```python
from build123d import *

# Parameters (mm, degrees)
SKETCH1_R           = 2.25
BOSS_EXTRUDE1_DEPTH = 2.6
SKETCH2_R           = 4.75
SKETCH2_R_2         = 2.5
BOSS_EXTRUDE2_DEPTH = 4.5
CHAMFER1_SIZE       = 0.75
SKETCH3_R           = 3.75
BOSS_EXTRUDE3_DEPTH = 3
CHAMFER2_SIZE       = 0.3
CHAMFER3_SIZE       = 0.5


with BuildPart() as part:
    # Sketch1 → Boss-Extrude1 (new body)
    with BuildSketch(Plane(origin=(0, 0, 0), x_dir=(0, 0, -1), z_dir=(1, 0, 0))):
        with BuildLine():
            Line((-21, -10), (6, -10))
            ThreePointArc((6, -10), (8.828427125, -8.828427125), (10, -6))
            Line((10, -6), (10, 19))
            ThreePointArc((10, 19), (8.828427125, 21.828427125), (6, 23))
            Line((6, 23), (-9.695652174, 23))
            ThreePointArc((-9.695652174, 23), (-11.354136506, 22.63997661), (-12.714074263, 21.62471486))
            Line((-12.714074263, 21.62471486), (-24.018422089, 8.62471486))
            ThreePointArc((-24.018422089, 8.62471486), (-24.746577662, 7.401126626), (-25, 6))
            Line((-25, 6), (-25, -6))
            ThreePointArc((-25, -6), (-23.828427125, -8.828427125), (-21, -10))
        make_face()
        with Locations((-15, 0)):
            Circle(SKETCH1_R, mode=Mode.SUBTRACT)
        with Locations((0, 17.25)):
            Circle(SKETCH1_R, mode=Mode.SUBTRACT)
        Circle(SKETCH1_R, mode=Mode.SUBTRACT)
    extrude(amount=BOSS_EXTRUDE1_DEPTH)

    # Sketch2 → Boss-Extrude2 (add)
    with BuildSketch(Plane.ZY):
        with Locations(Location((0, 17.25, 0), (0, 0, 180))):
            Circle(SKETCH2_R)
        with Locations((0, 17.25)):
            Circle(SKETCH2_R_2, mode=Mode.SUBTRACT)
    extrude(amount=BOSS_EXTRUDE2_DEPTH)

    # Chamfer1
    chamfer1_edges = [part.edges().sort_by_distance(p)[0] for p in [
        (-4.5, 17.25, 4.75),
    ]]
    chamfer(chamfer1_edges, length=CHAMFER1_SIZE)

    # Sketch3 → Boss-Extrude3 (add)
    with BuildSketch(Plane(origin=(2.6, 0, 0), x_dir=(0, 0, -1), z_dir=(1, 0, 0))):
        with BuildLine():
            Line((-21, -10), (6, -10))
            ThreePointArc((6, -10), (8.828427125, -8.828427125), (10, -6))
            Line((10, -6), (10, 19))
            ThreePointArc((10, 19), (8.828427125, 21.828427125), (6, 23))
            Line((6, 23), (-9.695652174, 23))
            ThreePointArc((-9.695652174, 23), (-11.354136506, 22.63997661), (-12.714074263, 21.62471486))
            Line((-12.714074263, 21.62471486), (-24.018422089, 8.62471486))
            ThreePointArc((-24.018422089, 8.62471486), (-24.746577662, 7.401126626), (-25, 6))
            Line((-25, 6), (-25, -6))
            ThreePointArc((-25, -6), (-23.828427125, -8.828427125), (-21, -10))
        make_face()
        with Locations((-15, 0)):
            Circle(SKETCH3_R, mode=Mode.SUBTRACT)
        Circle(SKETCH3_R, mode=Mode.SUBTRACT)
        Polygon((2.165063509, 21), (-2.165063509, 21), (-4.330127019, 17.25), (-2.165063509, 13.5), (2.165063509, 13.5), (4.330127019, 17.25), align=None, mode=Mode.SUBTRACT)
    extrude(amount=BOSS_EXTRUDE3_DEPTH)

    # Chamfer2
    chamfer2_edges = [part.edges().sort_by_distance(p)[0] for p in [
        (2.6, 0, 17.25),
        (2.6, 17.25, 2.25),
        (2.6, 0, 2.25),
        (2.6, 0, 3.75),
        (2.6, 0, 18.75),
        (2.6, 19.125, -3.247595264),
        (2.6, 21, 0),
        (2.6, 19.125, 3.247595264),
        (2.6, 15.375, 3.247595264),
        (2.6, 13.5, 0),
        (2.6, 15.375, -3.247595264),
    ]]
    chamfer(chamfer2_edges, length=CHAMFER2_SIZE)

    # Chamfer3
    chamfer3_edges = [part.edges().sort_by_distance(p)[0] for p in [
        (5.6, -8.828427125, 23.828427125),
        (5.6, -10, 7.5),
        (5.6, -8.828427125, -8.828427125),
        (5.6, 6.5, -10),
        (5.6, 21.828427125, -8.828427125),
        (5.6, 23, 1.847826087),
        (5.6, 22.63997661, 11.354136506),
        (5.6, 15.12471486, 18.366248176),
        (5.6, 7.401126626, 24.746577662),
        (5.6, 0, 25),
        (5.6, 0, 18.75),
        (5.6, 0, 3.75),
        (5.6, 19.125, -3.247595264),
        (5.6, 21, 0),
        (5.6, 19.125, 3.247595264),
        (5.6, 15.375, 3.247595264),
        (5.6, 13.5, 0),
        (5.6, 15.375, -3.247595264),
    ]]
    chamfer(chamfer3_edges, length=CHAMFER3_SIZE)


solid = part.part
```
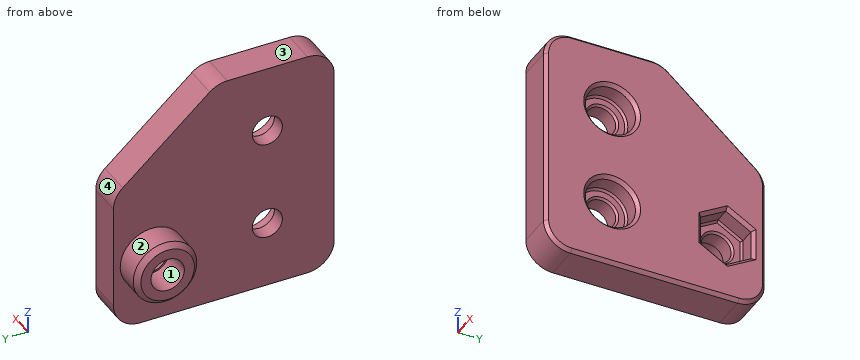
Part model, mm, in its own coordinate system. Face numbers are marked on the shaded views. Round coordinates to 2 decimals unless told otherwise and drop trailing zeros. Loops run counter-clockwise (first coordinate to the right, second up) from the corner with the lowest first, then second, coordinate; pieces in that order, holes last. Notation, with made-up numbers: (27.5, -1.5) -> (47.5, -1.5) arc R25 cw to (47.5, 34.5) -> close; hole circle Ø8 at (-31, -22.75). An arc over 180 degrees is marked (long way). Use a Markdown table: item, result.
1) Probe line 1 (Y direction, x = 0.9, z = 0); line 2 (Y direction, x = 0.75, z = -1); line 3 (X direction, y = 1.5, z = 20.5). List the from-to ranges inside material, lowest first. Write a range as [from, to].
The answers:
| item | result |
|---|---|
| line 1 | y = [-10, -2.25], [2.25, 15], [19.5, 23] |
| line 2 | y = [-10, -2.02], [2.02, 15.23], [19.27, 23] |
| line 3 | x = [0, 5.6] |
2) Cut at B-B, the plane x = 3.5. List the corners of the cut face in (y, z), and give its area (3 significant figures).
The answers:
| item | result |
|---|---|
| outline | (-10, -6) arc R4 ccw to (-6, -10) -> (19, -10) arc R4 ccw to (23, -6) -> (23, 9.7) arc R4 ccw to (21.62, 12.71) -> (8.62, 24.02) arc R4 ccw to (6, 25) -> (-6, 25) arc R4 ccw to (-10, 21) -> close; hole circle Ø7.5 at (0, 0); hole circle Ø7.5 at (0, 15); hole (13.5, -2.17) -> (17.25, -4.33) -> (21, -2.17) -> (21, 2.17) -> (17.25, 4.33) -> (13.5, 2.17) -> close |
| area | 902 mm2 |
3) Cut at D-D, the plane x = -1.25. List the corners of the cut face in (y, z), and give its area (3 significant figures).
The answers:
| item | result |
|---|---|
| outline | circle Ø9.5 at (17.25, 0); hole circle Ø5 at (17.25, 0) |
| area | 51.2 mm2 |
4) Drop flat-ended pins along their axis: pin 1 Ø2 at (y, z) = (0, -1) entering from +X; pin 2 Ø2 at (x, y) = (2, 16) entering from +Z; pin 3 Ø6 at (y, z) = (17.25, 0) entering from +X; pin 4 Ø7 at (y, z) = (0, 0) entering from +X. Give the stop position or say it passes through.
The answers:
| item | result |
|---|---|
| pin 1 | passes through |
| pin 2 | stops at z = 18.47 |
| pin 3 | stops at x = 2.6 |
| pin 4 | stops at x = 2.65 |
5) Pull direction Y, two halves, no side cores. Call the marked faces 1, 2, 3 and 4: pulls with the +Y half, pulls with the -Y half, needs draft (parallel to the pull), parting line crosses it, or undercut.
The answers:
| item | result |
|---|---|
| face 1 | undercut |
| face 2 | parting line crosses it |
| face 3 | needs draft |
| face 4 | pulls with the +Y half |
6) Cut at A-A, the plane y = 0. State how many separate pieces and enclosed holes the cut face has, and give its area (3 significant figures).
The answers:
| item | result |
|---|---|
| separate pieces | 3 |
| enclosed holes | 0 |
| area | 127 mm2 |
7) Cut at C-C, the plane z = 15. List the corners of the cut face in (x, y).
The answers:
| item | result |
|---|---|
| outline | (0, -10) -> (5.1, -10) -> (5.6, -9.5) -> (5.6, -4.25) -> (5.1, -3.75) -> (2.9, -3.75) -> (2.6, -3.45) -> (2.6, -2.55) -> (2.3, -2.25) -> (0, -2.25) -> close; (0, 2.25) -> (2.3, 2.25) -> (2.6, 2.55) -> (2.6, 3.45) -> (2.9, 3.75) -> (5.1, 3.75) -> (5.6, 4.25) -> (5.6, 18.23) -> (5.1, 19) -> (0, 19) -> close |
